```python
from build123d import *

# Parameters (mm, degrees)
BOSS_EXTRUDE1_DEPTH     = 12.7
SKETCH3_R               = 6.35
CUT_EXTRUDE1_DEPTH      = 76.134213245
BOSS_EXTRUDE2_DEPTH     = 12.7
SKETCH5_R               = 33.655
CUT_EXTRUDE2_DEPTH      = 126.483214241
BOSS_EXTRUDE3_START     = -6.35
SKETCH6_R               = 33.655
SKETCH6_R_2             = 20.955
BOSS_EXTRUDE3_DEPTH     = 6.35
CUT_EXTRUDE3_REACH      = 122.901
CUT_EXTRUDE3_END_RADIUS = 33.655
SKETCH7_R               = 3.175
CIRPATTERN1_COUNT       = 3
CUT_EXTRUDE4_DEPTH      = 112.134524666
FILLET1_R               = 3.175


with BuildPart() as part:
    # Sketch1 → Boss-Extrude1 (new body)
    with BuildSketch(Plane(origin=(0, 0, 0), x_dir=(1, 0, 0), z_dir=(0, 1, 0))):
        with BuildLine():
            Line((-57.15, 38.1), (57.15, 38.1))
            ThreePointArc((57.15, 38.1), (61.640128061, 36.240128061), (63.5, 31.75))
            Line((63.5, 31.75), (63.5, -31.75))
            ThreePointArc((63.5, -31.75), (61.640128061, -36.240128061), (57.15, -38.1))
            Line((57.15, -38.1), (-57.15, -38.1))
            ThreePointArc((-57.15, -38.1), (-61.640128061, -36.240128061), (-63.5, -31.75))
            Line((-63.5, -31.75), (-63.5, 31.75))
            ThreePointArc((-63.5, 31.75), (-61.640128061, 36.240128061), (-57.15, 38.1))
        make_face()
    extrude(amount=-BOSS_EXTRUDE1_DEPTH)

    # Sketch3 → Cut-Extrude1 (cut, through all)
    with BuildSketch(Plane.XZ.offset(12.7)):
        with Locations(Location((-50.8, 22.225, 0), (0, 0, 270))):
            Circle(SKETCH3_R)
        with Locations(Location((50.8, 22.225, 0), (0, 0, 90))):
            Circle(SKETCH3_R)
        with Locations(Location((0, -25.4, 0), (0, 0, 270))):
            Circle(SKETCH3_R)
    extrude(amount=-CUT_EXTRUDE1_DEPTH, mode=Mode.SUBTRACT)

    # Sketch2 → Boss-Extrude2 (add, symmetric)
    with BuildSketch(Plane.XY):
        with BuildLine():
            Line((-41.91, -12.7), (-40.947154642, -55.530506915))
            ThreePointArc((-40.947154642, -55.530506915), (0, -95.5675), (40.947154642, -55.530506915))
            Line((40.947154642, -55.530506915), (41.91, -12.7))
            Line((41.91, -12.7), (-41.91, -12.7))
        make_face()
    extrude(amount=BOSS_EXTRUDE2_DEPTH, both=True)

    # Sketch5 → Cut-Extrude2 (cut, through all)
    with BuildSketch(Plane.XY.offset(12.7)):
        with Locations((0, -54.61)):
            Circle(SKETCH5_R)
    extrude(amount=-CUT_EXTRUDE2_DEPTH, mode=Mode.SUBTRACT)

    # Sketch6 → Boss-Extrude3 (add)
    with BuildSketch(Plane(origin=(0, 0, -12.7), x_dir=(-1, 0, 0), z_dir=(0, 0, -1)).offset(BOSS_EXTRUDE3_START)):
        with Locations(Location((0, -54.61, 0), (0, 0, 180))):
            Circle(SKETCH6_R)
        with Locations((0, -54.61)):
            Circle(SKETCH6_R_2, mode=Mode.SUBTRACT)
    extrude(amount=BOSS_EXTRUDE3_DEPTH)

    # Cut-Extrude3: up to this cylinder (the profile starts outside it)
    cut_extrude3_end = Plane(origin=(0, -54.61, 3.175), z_dir=(0, 0, 1)) * Cylinder(CUT_EXTRUDE3_END_RADIUS, 314.112, mode=Mode.PRIVATE)
    # Sketch7 → Cut-Extrude3 (cut, up to the surface)
    with BuildSketch(Plane(origin=(0, 0, 0), x_dir=(1, 0, 0), z_dir=(0, 1, 0)), mode=Mode.PRIVATE) as cut_extrude3_sk1:
        with Locations(Location((0, -3.175, 0), (0, 0, 270))):
            Circle(SKETCH7_R)
    cut_extrude3_tool1 = extrude(cut_extrude3_sk1.sketch, amount=-CUT_EXTRUDE3_REACH, mode=Mode.PRIVATE) - cut_extrude3_end
    cut_extrude3 = cut_extrude3_tool1.solids().sort_by_distance((0, 0, 3.175))[0]
    add(cut_extrude3, mode=Mode.SUBTRACT)

    # CirPattern1: Cut-Extrude3 ×3 about axis
    cirpattern1_axis = Axis((0, -54.61, 12.7), (0, 0, 1))
    for i in range(1, CIRPATTERN1_COUNT):
        add(cut_extrude3.rotate(cirpattern1_axis, i * 360 / CIRPATTERN1_COUNT), mode=Mode.SUBTRACT)

    # Sketch8 → Cut-Extrude4 (cut, through all)
    with BuildSketch(Plane.XZ.offset(12.7)):
        with BuildLine():
            Line((-63.5, 0), (-25.4, -38.1))
            Line((-25.4, -38.1), (-57.15, -38.1))
            ThreePointArc((-57.15, -38.1), (-61.640128061, -36.240128061), (-63.5, -31.75))
            Line((-63.5, -31.75), (-63.5, 0))
        make_face()
        with BuildLine():
            Line((57.15, -38.1), (25.4, -38.1))
            Line((25.4, -38.1), (63.5, 0))
            Line((63.5, 0), (63.5, -31.75))
            ThreePointArc((63.5, -31.75), (61.640128061, -36.240128061), (57.15, -38.1))
        make_face()
    extrude(amount=-CUT_EXTRUDE4_DEPTH, mode=Mode.SUBTRACT)

    # Fillet1
    fillet1_edges = [part.edges().sort_by_distance(p)[0] for p in [
        (0, -12.7, -12.7),
        (41.91, -12.7, 0),
        (-41.91, -12.7, 0),
        (0, -12.7, 12.7),
        (-63.5, -6.35, 0),
        (-25.4, -6.35, -38.1),
        (25.4, -6.35, -38.1),
        (63.5, -6.35, 0),
    ]]
    fillet(fillet1_edges, radius=FILLET1_R)


solid = part.part
```
CAD build for the part. Positions are in the model's coordinates, mm. A direction names the side the tool comes from. Coordinates: 2 decimals unless noted, no trailing zeros. Order: outer loops, then holes, each group sorted by start corner. A loop starts at its lowest first (then second) coordinate and runs counter-clockwise, first axis right, second up. Notation, with made-up numbers: M 61.5,22.5 L 71.5,22.5 A23 ccw 71.5,55.5 Z; hole C -33,-39.5 d3. An arc over 180 degrees is marked long. Answer as CSV lines item,"result".
1) Cut at B-B (x = 50.8). List the corners of the cut face in (y, z) (3 decimals).
Verdict:
outline,"M -12.7,-12.7 L 0,-12.7 L 0,15.875 L -12.7,15.875 Z; M -12.7,28.575 L 0,28.575 L 0,38.1 L -12.7,38.1 Z"
2) Flat gauge pins, fed straight in: P1, Ø2, axis at x = 40, z = -16.5, coming from the -Y side; P2, Ø14.5, axis at x = 0, z = -25.4, coming from the +Y side; P3, Ø24, axis at x = -18.5, y = -61, coming from the +Z side; P4, Ø5, axis at x = -45.5, z = 0, coming from the -Y side. Where does each tip first touch, or does it go through?
Verdict:
P1,"y = -12.72"
P2,"y = 0"
P3,"z = -6.35"
P4,"y = -13.42"
3) Mould opens along Y. For faces 1 (the cylindrical face through (2.728, -33.833, -9.481)), 2 (the flat face through (-44.7, -6.4, -18.8)), 3 (the cylindrical face through (42.8, -13.6, -0.2)), 4 (the flat face through (14.5, -70, -6.35)) say: released by +Y, released by -Y, zero draft, split by the parting line, or undercut.
Verdict:
face 1,"undercut"
face 2,"zero draft"
face 3,"released by -Y"
face 4,"undercut"
4) Cut at D-D (y = -43). List the corners of the cut face in (x, z), then the cut area to 3 significant figures.
Verdict:
outline,"M -41.23,-12.7 L -17.44,-12.7 L -17.44,-6.35 L -31.59,-6.35 L -31.59,12.7 L -41.23,12.7 Z; M 17.44,-12.7 L 41.23,-12.7 L 41.23,12.7 L 31.59,12.7 L 31.59,-6.35 L 17.44,-6.35 Z"
area,"669 mm2"
5) 3-axis set-ups, long thin cutter, end or side, ignore diameter. For faces 5 (the cylindrical face through (33.696, -70.812, 4.64)), 6 (the cylindrical face through (0.954, -10.407, 6.203)), 7 (the flat face through (-1, -30, -12.7)), 8 (the flat face through (-1, -20, 12.7)): which of +Z, -Z, +X, -X, +Y, -Y reach the whole face in a straight line?
Verdict:
face 5,"none"
face 6,"+Y"
face 7,"-Z, +X, -X, -Y"
face 8,"+Z, +X, -X, -Y"
6) Drill centre lines: L1, parallel to Y at x = -1, z = -4; L2, parallel to Y at x = -20, z = -17; L3, parallel to Z at x = 22.5, y = -50.5. Where is each one in solid material? Low to high. Write a range as from..to.
Verdict:
L1,"-95.56..-88.25, -20.97..0"
L2,"-12.7..0"
L3,"-12.7..-6.35"
7) Cut at A-A (x = 0). Give the number of separate pieces and of enclosed holes in the cut face, then the cut area to 3 significant figures.
Verdict:
separate pieces,"4"
enclosed holes,"0"
area,"1,230 mm2"
8) Cut at C-C (z = -25.4). List the corners of the cut face in (x, y), then the cut area to 3 significant figures.
Verdict:
outline,"M -38.1,-12.7 L -6.35,-12.7 L -6.35,0 L -38.1,0 Z; M 6.35,-12.7 L 38.1,-12.7 L 38.1,0 L 6.35,0 Z"
area,"806 mm2"
